from build123d import *

# Parameters (mm, degrees)
SKETCH1_W           = 30
SKETCH1_H           = 30
BOSS_EXTRUDE1_DEPTH = 118
SKETCH2_R           = 8.5
CUT_EXTRUDE1_DEPTH  = 19
SKETCH3_R           = 9
CUT_EXTRUDE2_DEPTH  = 26
SKETCH4_R           = 10
CUT_EXTRUDE3_DEPTH  = 32
SKETCH5_R           = 8.5
CUT_EXTRUDE4_DEPTH  = 44
FILLET3_R           = 10
FILLET4_R           = 3
FILLET5_R           = 3
FILLET6_R           = 3
FILLET7_R           = 3
FILLET8_R           = 3


with BuildPart() as part:
    # Sketch1 → Boss-Extrude1 (new body)
    with BuildSketch(Plane(origin=(0, 0, 0), x_dir=(0, 0, -1), z_dir=(1, 0, 0))):
        Rectangle(SKETCH1_W, SKETCH1_H)
    extrude(amount=BOSS_EXTRUDE1_DEPTH)

    # Sketch2 → Cut-Extrude1 (cut)
    with BuildSketch(Plane(origin=(118, 0, 0), x_dir=(0, 0, -1), z_dir=(1, 0, 0))):
        Circle(SKETCH2_R)
    extrude(amount=-CUT_EXTRUDE1_DEPTH, mode=Mode.SUBTRACT)

    # Sketch3 → Cut-Extrude2 (cut)
    with BuildSketch(Plane(origin=(99, 0, 0), x_dir=(0, 0, -1), z_dir=(1, 0, 0))):
        Circle(SKETCH3_R)
    extrude(amount=-CUT_EXTRUDE2_DEPTH, mode=Mode.SUBTRACT)

    # Sketch4 → Cut-Extrude3 (cut)
    with BuildSketch(Plane(origin=(73, 0, 0), x_dir=(0, 0, -1), z_dir=(1, 0, 0))):
        Circle(SKETCH4_R)
    extrude(amount=-CUT_EXTRUDE3_DEPTH, mode=Mode.SUBTRACT)

    # Sketch5 → Cut-Extrude4 (cut)
    with BuildSketch(Plane(origin=(41, 0, 0), x_dir=(0, 0, -1), z_dir=(1, 0, 0))):
        Circle(SKETCH5_R)
    extrude(amount=-CUT_EXTRUDE4_DEPTH, mode=Mode.SUBTRACT)

    # Fillet3
    # the kernel refuses this fillet: 10 mm, written as the material it takes off along each edge
    with BuildSketch(Plane(origin=(41, 0, 0), x_dir=(0, 0, -1), z_dir=(0, -1, 0))) as fillet3_piece_1:
        with BuildLine():
            CenterArc((18.5, -5.267826876), FILLET3_R, 148.211669383, 31.788330617)
            Line((10, 0), (9.83, 0.105356538))
            ThreePointArc((9.83, 0.105356538), (9.25, 0.2), (8.5, 0.2))
            Line((8.5, 0.2), (8.3, 0))
            Line((8.3, 0), (8.3, -5.267826876))
            Line((8.3, -5.267826876), (8.5, -5.267826876))
        make_face()
    revolve(axis=Axis((41, 0, 0), (1, 0, 0)), mode=Mode.SUBTRACT)

    # Fillet4
    fillet4_edges = [part.edges().sort_by_distance(p)[0] for p in [
        (41, 0, 10),
    ]]
    fillet(fillet4_edges, radius=FILLET4_R)

    # Fillet5
    # the kernel refuses this fillet: 3 mm, written as the material it takes off along each edge
    with BuildSketch(Plane(origin=(73, 0, 0), x_dir=(0, 0, -1), z_dir=(0, -1, 0))) as fillet5_piece_1:
        with BuildLine():
            CenterArc((12, 2.236067977), FILLET5_R, 180, 48.189685104)
            Line((9, 2.236067977), (8.94, 2.236067977))
            Line((8.94, 2.236067977), (8.94, 0))
            Line((8.94, 0), (9, -0.06))
            ThreePointArc((9, -0.06), (9.5, -0.06), (9.96, -0.04472136))
            Line((9.96, -0.04472136), (10, 0))
        make_face()
    revolve(axis=Axis((73, 0, 0), (1, 0, 0)), mode=Mode.SUBTRACT)

    # Fillet6
    fillet6_edges = [part.edges().sort_by_distance(p)[0] for p in [
        (73, 0, 10),
    ]]
    fillet(fillet6_edges, radius=FILLET6_R)

    # Fillet7
    # the kernel refuses this fillet: 3 mm, written as the material it takes off along each edge
    with BuildSketch(Plane(origin=(99, 0, 0), x_dir=(0, 0, -1), z_dir=(0, -1, 0))) as fillet7_piece_1:
        with BuildLine():
            CenterArc((11.5, 1.658312395), FILLET7_R, 180, 33.557309762)
            Line((8.5, 1.658312395), (8.44, 1.658312395))
            Line((8.44, 1.658312395), (8.44, 0))
            Line((8.44, 0), (8.5, -0.06))
            ThreePointArc((8.5, -0.06), (8.75, -0.06), (8.95, -0.033166248))
            Line((8.95, -0.033166248), (9, 0))
        make_face()
    revolve(axis=Axis((99, 0, 0), (1, 0, 0)), mode=Mode.SUBTRACT)

    # Fillet8
    fillet8_edges = [part.edges().sort_by_distance(p)[0] for p in [
        (99, 0, 9),
    ]]
    fillet(fillet8_edges, radius=FILLET8_R)


solid = part.part
Geometry check sheet. Reference: the model listing, model coordinates, mm. A direction names the side the tool comes from. Give positions to 0.01 mm unless a question says otherwise; leave off trailing zeros. Loops run counter-clockwise (first coordinate to the right, second up) from the corner with the lowest first, then second, coordinate; pieces in that order, holes last.
(1) Section check B-B on x = 104.5. Record the cut outline in (y, z).
From the geometry:
outline: (-15, -15) - (15, -15) - (15, 15) - (-15, 15) - close; hole circle Ø17 at (0, 0)
(2) Depth check by flat-ended pin: pin 1 Ø4 at (y, z) = (1, 9.5) entering from -X; pin 2 Ø10 at (y, z) = (0, 0) entering from +X. Enter the tip coordinate at first touch or a pass-through.
From the geometry:
pin 1: stops at x = 0
pin 2: passes through
(3) Set-up check for faces 4 (the flat face through (58, 0, 15)), 5 (the cylindrical face through (86.909, -3.447, -8.314)): record each of +Z, -Z, +X, -X, +Y, -Y from which the full face is reachable in a straight line by a thin tool's end or side.
From the geometry:
face 4: +Z, +X, -X, +Y, -Y
face 5: none
(4) Section check A-A on x = 48. Record the cut outline in (y, z), then the cut area to 3 significant figures.
From the geometry:
outline: (-15, -15) - (15, -15) - (15, 15) - (-15, 15) - close; hole circle Ø20 at (0, 0)
area: 586 mm2
(5) Release check for a two-part mould opening along Z. For faces 1 (the cylindrical face through (57.07, -9.76, 2.17)), 2 (the flat face through (58, 0, -15)), 3 (the flat face through (118, 7, 7)) record: released by +Z, released by -Z, zero draft, split by the parting line, or undercut.
From the geometry:
face 1: undercut
face 2: released by -Z
face 3: zero draft
(6) Thickness scan on L1, parallel to Y at x = 7.5, z = 0; L2, parallel to Y at x = 58, z = 0. Record the ranges inside material, lowest first.
From the geometry:
L1: y = -15 to -8.5, 8.5 to 15
L2: y = -15 to -10, 10 to 15
